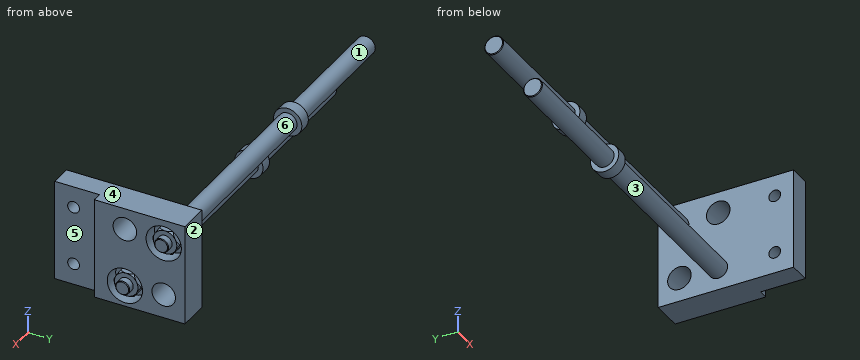
from build123d import *

# Parameters (mm, degrees)
BOSS_EXTRUDE1_DEPTH      = 10.2
BOSS_EXTRUDE1_DEPTH_BACK = 32.8
SKETCH1_W                = 13
SKETCH1_H                = 57.5
CUT_EXTRUDE1_DEPTH       = 60.975745097
CUT_EXTRUDE1_DEPTH_BACK  = 60.975745097
SKETCH3_W                = 4
SKETCH3_H                = 19
SKETCH4_R                = 7.5
CUT_EXTRUDE2_DEPTH       = 6.5
BOSS_EXTRUDE2_DEPTH      = 5.5
SKETCH8_R                = 3
BOSS_EXTRUDE3_DEPTH      = 3
CHAMFER1_SIZE            = 0.3
SKETCH10_R               = 5
CUT_EXTRUDE3_DEPTH       = 61.44079748
SKETCH9_R                = 4
BOSS_EXTRUDE4_DEPTH      = 143
CHAMFER2_SIZE            = 0.3
SKETCH11_R               = 2.5
CUT_EXTRUDE4_DEPTH       = 155.522134337
SKETCH12_R               = 6
BOSS_EXTRUDE5_DEPTH      = 5


with BuildPart() as part:
    # Sketch1 → Boss-Extrude1 (new, two sides: drawn at the far end of the back side and taken through both)
    with BuildSketch(Plane.XY.offset(-BOSS_EXTRUDE1_DEPTH_BACK)):
        with Locations((6.5, -19.75)):
            Rectangle(SKETCH1_W, SKETCH1_H)
    extrude(amount=BOSS_EXTRUDE1_DEPTH + BOSS_EXTRUDE1_DEPTH_BACK)

    # Sketch3 → Cut-Extrude1 (cut, two sides: drawn at the far end of the back side and taken through both)
    with BuildSketch(Plane.XY.offset(-CUT_EXTRUDE1_DEPTH_BACK)):
        with Locations((11, -39)):
            Rectangle(SKETCH3_W, SKETCH3_H)
    extrude(amount=CUT_EXTRUDE1_DEPTH + CUT_EXTRUDE1_DEPTH_BACK, mode=Mode.SUBTRACT)

    # Sketch4 → Cut-Extrude2 (cut)
    with BuildSketch(Plane(origin=(13, 0, 0), x_dir=(0, 0, -1), z_dir=(1, 0, 0))):
        with Locations(Location((0, 0, 0), (0, 0, 90))):
            Circle(SKETCH4_R)
        with Locations(Location((23.8, -16.5, 0), (0, 0, 90))):
            Circle(SKETCH4_R)
    extrude(amount=-CUT_EXTRUDE2_DEPTH, mode=Mode.SUBTRACT)

    # Sketch5 → Boss-Extrude2 (add)
    with BuildSketch(Plane(origin=(6.5, 0, 0), x_dir=(0, 0, -1), z_dir=(1, 0, 0))):
        Polygon((0, 5.773502692), (-5, 2.886751346), (-5, -2.886751346), (0, -5.773502692), (5, -2.886751346), (5, 2.886751346), align=None)
        Polygon((23.8, -10.726497308), (18.8, -13.613248654), (18.8, -19.386751346), (23.8, -22.273502692), (28.8, -19.386751346), (28.8, -13.613248654), align=None)
    extrude(amount=BOSS_EXTRUDE2_DEPTH)

    # Sketch6 → Cut-Revolve1 (revolve, cut)
    with BuildSketch(Plane(origin=(0, 0, 0), x_dir=(-1, 0, 0), z_dir=(0, 0, -1)), mode=Mode.PRIVATE) as cut_revolve1_sk:
        Polygon((-12, 5.773502692), (-12, 4.992217065), (-11, 5.773502692), align=None)
    revolve(cut_revolve1_sk.sketch.rotate(Axis((6.5, 0, 0), (1, 0, 0)), 180), axis=Axis((6.5, 0, 0), (1, 0, 0)), mode=Mode.SUBTRACT)

    # Sketch7 → Cut-Revolve2 (revolve, cut)
    with BuildSketch(Plane(origin=(0, 0, -23.8), x_dir=(-1, 0, 0), z_dir=(0, 0, -1)), mode=Mode.PRIVATE) as cut_revolve2_sk:
        Polygon((-11, -10.726497308), (-12, -10.726497308), (-12, -11.507782935), align=None)
    revolve(cut_revolve2_sk.sketch.rotate(Axis((6.5, -16.5, -23.8), (1, 0, 0)), 90), axis=Axis((6.5, -16.5, -23.8), (1, 0, 0)), mode=Mode.SUBTRACT)

    # Sketch8 → Boss-Extrude3 (add)
    with BuildSketch(Plane(origin=(12, 0, 0), x_dir=(0, 0, -1), z_dir=(1, 0, 0))):
        with Locations(Location((0, 0, 0), (0, 0, 90))):
            Circle(SKETCH8_R)
        with Locations(Location((23.8, -16.5, 0), (0, 0, 90))):
            Circle(SKETCH8_R)
    extrude(amount=BOSS_EXTRUDE3_DEPTH)

    # Chamfer1
    chamfer1_edges = [part.edges().sort_by_distance(p)[0] for p in [
        (15, -3, 0),
        (15, -19.5, -23.8),
    ]]
    chamfer(chamfer1_edges, length=CHAMFER1_SIZE)

    # Sketch10 → Cut-Extrude3 (cut, through all)
    with BuildSketch(Plane(origin=(0, 0, 0), x_dir=(0, 0, -1), z_dir=(1, 0, 0))):
        with Locations(Location((22.6, 0, 0), (0, 0, 90))):
            Circle(SKETCH10_R)
        with Locations(Location((-1.2, -16.5, 0), (0, 0, 90))):
            Circle(SKETCH10_R)
    extrude(amount=CUT_EXTRUDE3_DEPTH, mode=Mode.SUBTRACT)

    # Sketch9 → Boss-Extrude4 (add)
    with BuildSketch(Plane(origin=(0, 0, 0), x_dir=(0, 0, -1), z_dir=(1, 0, 0))):
        with Locations((23.8, -16.5)):
            Circle(SKETCH9_R)
        Circle(SKETCH9_R)
    extrude(amount=-BOSS_EXTRUDE4_DEPTH)

    # Chamfer2
    chamfer2_edges = [part.edges().sort_by_distance(p)[0] for p in [
        (-143, -16.5, -19.8),
        (-143, 0, 4),
    ]]
    chamfer(chamfer2_edges, length=CHAMFER2_SIZE)

    # Sketch11 → Cut-Extrude4 (cut, through all)
    with BuildSketch(Plane(origin=(0, 0, 0), x_dir=(0, 0, -1), z_dir=(1, 0, 0))):
        with Locations(Location((-1.2, -40.5, 0), (0, 0, 270))):
            Circle(SKETCH11_R)
        with Locations(Location((23.8, -40.5, 0), (0, 0, 270))):
            Circle(SKETCH11_R)
    extrude(amount=CUT_EXTRUDE4_DEPTH, mode=Mode.SUBTRACT)

    # Sketch12 → Boss-Extrude5 (add)
    with BuildSketch(Plane(origin=(-87.5, 0, 0), x_dir=(0, 0, -1), z_dir=(1, 0, 0))):
        Circle(SKETCH12_R)
        with Locations((23.8, -16.5)):
            Circle(SKETCH12_R)
    extrude(amount=BOSS_EXTRUDE5_DEPTH)


solid = part.part
Can you work these out from the model? Positions are in its coordinate system, mm. Face numbers are marked on the shaded views. A direction names the side the tool comes from. Give positions to 0.01 mm unless a question says otherwise; leave off trailing zeros. Order: outer loops, then holes, each group sorted by start corner. A loop starts at its lowest first (then second) coordinate and runs counter-clockwise, first axis right, second up. Notation, with made-up numbers: M -31,4.5 L 4,4.5 A20 cw 4,26.5 Z; hole C -30,49.5 d8. An arc over 180 degrees is marked long. Use a Markdown table: item, result. Add a question column.
Item 1: For the marked faces 1, 2 and 3, which set-ups out of +Z, -Z, +X, -X, +Y, -Y let a thin tool reach every point of the face, with its end or its side?
Item 2: If I drill on L1, parallel to Z at x = 9.75, y = -16.5; L2, parallel to Z at x = 4.5, y = 0; L3, parallel to X at y = -36, z = -25.5, over which ranges is the centre line in solid material (lowest first)? Write a range as [from, to].
Item 3: Will these pins go through, and if not, where does the flat tip stop? pin 1 (12 mm diameter, centred on x = -17, z = -25, fed in from -Y); pin 2 (1 mm diameter, centred on x = -101.5, y = -2.5, fed in from -Z); pin 3 (6 mm diameter, centred on y = -40.5, z = -23.8, fed in from -X).
Item 4: Suppose I cut it at C-C (x = -57.5). List the corners of the cut face in (y, z) for me.
Item 5: We'd pull the mould along X, two halves only. Please class the marked faces 4, 5 and 6: +X half, -X half, draft (parallel to the pull), parting line (faces both ways), or undercut.
Item 6: Suppose I cut it at A-A (y = -40.5). List the corners of the cut face in (x, z) for me, then the cut area to 3 significant figures.
Item 7: Suppose I cut it at D-D (y = -33). List the corners of the cut face in (x, z) for me.
Item 8: Suppose I cut it at B-B (x = 3). List the corners of the cut face in (y, z) for me, then the cut area to 3 significant figures.
Answer sheet:
| question | item | result |
|---|---|---|
| 1 | face 1 | -X |
| 1 | face 2 | +Z, -Z, +X, -X, +Y |
| 1 | face 3 | none |
| 2 | L1 | z = [-32.8, -31.3], [-28.8, -18.8], [-16.3, -3.8], [6.2, 10.2] |
| 2 | L2 | z = [-32.8, -27.6], [-17.6, 10.2] |
| 2 | L3 | x = [0, 9] |
| 3 | pin 1 | stops at y = -20.5 |
| 3 | pin 2 | stops at z = -3.46 |
| 3 | pin 3 | stops at x = 0 |
| 4 | outline | C -16.5,-23.8 d8; C 0,0 d8 |
| 5 | face 4 | draft |
| 5 | face 5 | +X half |
| 5 | face 6 | undercut |
| 6 | outline | M 0,-32.8 L 9,-32.8 L 9,-26.3 L 0,-26.3 Z; M 0,-21.3 L 9,-21.3 L 9,-1.3 L 0,-1.3 Z; M 0,3.7 L 9,3.7 L 9,10.2 L 0,10.2 Z |
| 6 | area | 297 mm² |
| 7 | outline | M 0,-32.8 L 9,-32.8 L 9,10.2 L 0,10.2 Z |
| 8 | outline | M -48.5,-32.8 L 9,-32.8 L 9,10.2 L -48.5,10.2 Z; hole C -40.5,-23.8 d5; hole C -40.5,1.2 d5; hole C -16.5,1.2 d10; hole C 0,-22.6 d10 |
| 8 | area | 2,280 mm² |
